Design review of the part built by this model. Coordinates are the model's own, in mm. Face numbers are marked on the shaded views. Coordinates: 2 decimals unless noted, no trailing zeros. Loops run counter-clockwise (first coordinate to the right, second up) from the corner with the lowest first, then second, coordinate; pieces in that order, holes last. Notation, with made-up numbers: M -39.75,40 L -18.75,40 A23 cw -18.75,73 Z; hole C -23.75,-23 d3. An arc over 180 degrees is marked long. Put each result on its own line as item: value. Start each with the question number.
(1) The part is to be moulded in two halves that separate along X. For the marked faces 1, 2, 3 and 4, say which applies: +X half, -X half, draft (parallel to the pull), parting line (faces both ways), or undercut.
(2) Take a section at D-D, the plane x = 45. Give the boundary of the cut face in (y, z).
(3) For probe 1 along Z at (x, y) = (-31, 16); probe 2 along X at (y, z) = (29, 1.5); probe 3 along X at (y, z) = (6, -2), list the stretches that pass through material, from the lowest coordinate up. Write a range as [from, to].
(4) Take a section at B-B, the plane y = 31. Give the boundary of the cut face in (x, z), then the cut area to 3 significant figures.
(5) Take a section at C-C, the plane x = 31.75. Give the boundary of the cut face in (y, z).
(6) Take a section at A-A, the plane z = 0. Give the boundary of the cut face in (x, y).
```python
from build123d import *

# Parameters (mm, degrees)
F0_W     = 127
F0_H     = 127
F0_R     = 22.86
F1_DEPTH = 33.0962


with BuildPart() as f1:
    # F0 (on Front) → F1 (new body)
    with BuildSketch(Plane.XZ):
        Rectangle(F0_W, F0_H)
        with Locations((-31.75, 0)):
            Circle(F0_R, mode=Mode.SUBTRACT)
        with Locations((31.75, 0)):
            Circle(F0_R, mode=Mode.SUBTRACT)
    extrude(amount=-F1_DEPTH)


solid = f1.part
```
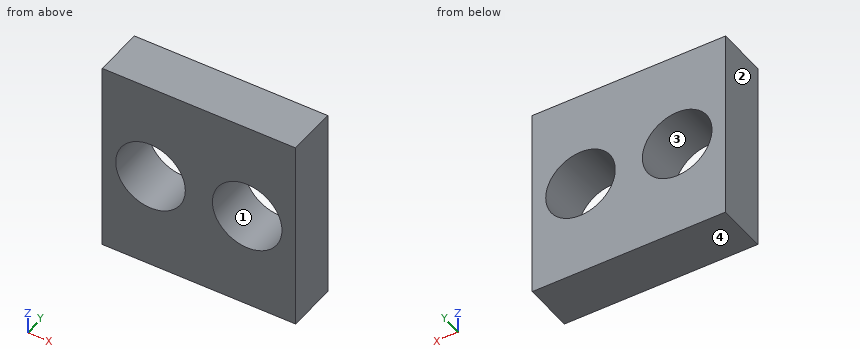
Computed values:
1. face 1: undercut
1. face 2: -X half
1. face 3: undercut
1. face 4: draft
2. outline: M 0,-63.5 L 33.1,-63.5 L 33.1,-18.63 L 0,-18.63 Z; M 0,18.63 L 33.1,18.63 L 33.1,63.5 L 0,63.5 Z
3. probe 1: z = [-63.5, -22.85], [22.85, 63.5]
3. probe 2: x = [-63.5, -54.56], [-8.94, 8.94], [54.56, 63.5]
3. probe 3: x = [-63.5, -54.52], [-8.98, 8.98], [54.52, 63.5]
4. outline: M -63.5,-63.5 L 63.5,-63.5 L 63.5,63.5 L -63.5,63.5 Z; hole C -31.75,0 d45.72; hole C 31.75,0 d45.72
4. area: 12,800 mm^2
5. outline: M 0,-63.5 L 33.1,-63.5 L 33.1,-22.86 L 0,-22.86 Z; M 0,22.86 L 33.1,22.86 L 33.1,63.5 L 0,63.5 Z
6. outline: M -63.5,0 L -54.61,0 L -54.61,33.1 L -63.5,33.1 Z; M -8.89,0 L 8.89,0 L 8.89,33.1 L -8.89,33.1 Z; M 54.61,0 L 63.5,0 L 63.5,33.1 L 54.61,33.1 Z
